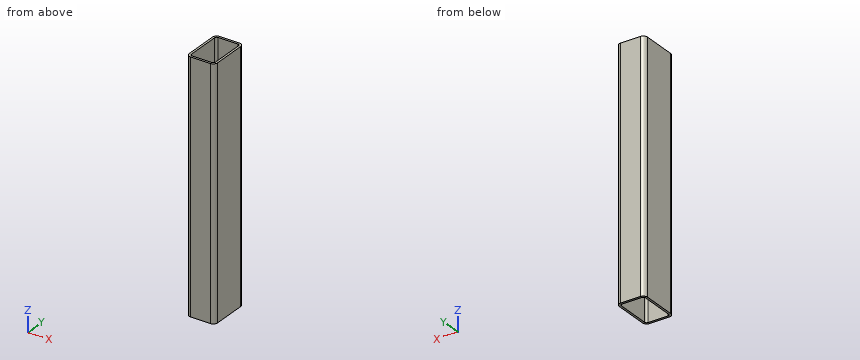
Autodesk Inventor part; units mm, degrees
ref_plane "Start Plane" through (0, 0, 40) normal (0, 0, 1) x (1, 0, 0)
ref_plane "End Plane" through (0, 0, 387) normal (0, 0, 1) x (1, 0, 0)
ref_plane "YZ Plane" through (0, 0, 0) normal (1, 0, 0) x (0, 1, 0)
ref_plane "Start Plane" through (0, 0, 40) normal (0, 0, 1) x (1, 0, 0)
ref_plane "End Plane" through (0, 0, 387) normal (0, 0, 1) x (1, 0, 0)
sketch "Sketch" plane through (0, 0, 0) normal (0, 0, 1) x (1, 0, 0)
  line L0 (-20, -24) -> (-20, 24)
  line L1 (-14, 30) -> (14, 30)
  line L2 (20, 24) -> (20, -24)
  line L3 (14, -30) -> (-14, -30)
  arc A0 (-20, -24) -> (-14, -30) centre (-14, -24) ccw
  arc A1 (20, 24) -> (14, 30) centre (14, 24) ccw
  arc A2 (-14, 30) -> (-20, 24) centre (-14, 24) ccw
  arc A3 (14, -30) -> (20, -24) centre (14, -24) ccw
  arc A4 (-14, 27) -> (-17, 24) centre (-14, 24) ccw
  line L4 (-14, 27) -> (14, 27)
  arc A5 (17, 24) -> (14, 27) centre (14, 24) ccw
  line L5 (17, 24) -> (17, -24)
  arc A6 (14, -27) -> (17, -24) centre (14, -24) ccw
  line L6 (14, -27) -> (-14, -27)
  arc A7 (-17, -24) -> (-14, -27) centre (-14, -24) ccw
  line L7 (-17, -24) -> (-17, 24)
  line L8 (0, 43.7397) -> (0, -43.7397) construction
  line L9 (-29.7397, 0) -> (29.7397, 0) construction
  dimension "d7" = 6
  dimension "d9" = 40
  dimension "d11" = 60
  dimension "d12" = 3
  dimension "d15" = 20
  dimension "d16" = 30
extrude "Body" add sketch "Sketch" along normal up to surface (347 mm away) from surface at 40
sketch "Sketch3" plane through (0, 0, 0) normal (0, 0, 1) x (1, 0, 0)
  line L0 (0, 0) -> (10, 0)
ref_plane "Work Plane3" through (0, 0, 0) normal (0, -1, 0) x (1, 0, 0)
sketch "Sketch4" plane through (0, 0, 0) normal (0, -1, 0) x (1, 0, 0)
  line L0 (-2, 40) -> (12, 40)
  line L1 (-2, 387) -> (12, 387)
  dimension "d18" = 347
equation "\"d7\" = G_IR"
equation "\"d9\" = G_W"
equation "\"d11\" = G_H"
equation "\"d12\" = G_T"
equation "\"d15\" = 0.5 * d9"
equation "\"d16\" = 0.5 * d11"
equation "\"d3\" = G_L"
equation "\"G_W\" = 40"
equation "\"G_H\" = 60"
equation "\"G_T\" = 3"
equation "\"G_IR\" = 6"
equation "\"G_L\" = d18"
equation "\"d14\" = G_OFFSET_END + B_L"
equation "\"B_L\" = 407"
properties part number "ISO 4019 - 60x40x3 - 347" material "Steel, Mild"
Input: part model. Units: mm. Frame: model coordinates. Give positions to 0.01 mm unless a question says otherwise; leave off trailing zeros. Order: outer loops, then holes, each group sorted by start corner. A loop starts at its lowest first (then second) coordinate and runs counter-clockwise, first axis right, second up. Notation, with made-up numbers: (-16.75, -32.5) - (-6.75, -32.5) arc R19 ccw to (-6.75, -21.5) - close; hole circle Ø6 at (17.5, 23.5). An arc over 180 degrees is marked (long way). Write each question's results on one line, items separated by ' | '.
Item 1: Section B-B (z = 346). Return loops of the section in (x, y).
A:
outline: (-20, -24) arc R6 ccw to (-14, -30) - (14, -30) arc R6 ccw to (20, -24) - (20, 24) arc R6 ccw to (14, 30) - (-14, 30) arc R6 ccw to (-20, 24) - close; hole (-17, -24) arc R3 ccw to (-14, -27) - (14, -27) arc R3 ccw to (17, -24) - (17, 24) arc R3 ccw to (14, 27) - (-14, 27) arc R3 ccw to (-17, 24) - close
Item 2: Section A-A (x = 2). Return loops of the section in (y, z).
A:
outline: (-30, 40) - (-27, 40) - (-27, 387) - (-30, 387) - close; (27, 40) - (30, 40) - (30, 387) - (27, 387) - close
Item 3: Section C-C (y = -14). Return loops of the section in (x, z).
A:
outline: (-20, 40) - (-17, 40) - (-17, 387) - (-20, 387) - close; (17, 40) - (20, 40) - (20, 387) - (17, 387) - close
Item 4: Material intervals for line 1 along Y through (x, z) = (-13, 340); line 2 along X through (y, z) = (-12, 335); line 3 along Y through (x, z) = (-16, 371.5), sorted ascending.
A:
line 1: y = -30 to -27, 27 to 30 | line 2: x = -20 to -17, 17 to 20 | line 3: y = -29.66 to -26.24, 26.24 to 29.66
